```python
from build123d import *

# Parameters (mm, degrees)
EXTRUDE_1_DEPTH     = 0.45
CUT_EXTRUDE_1_DEPTH = 5
SKETCH_4_R          = 0.75
SKETCH_4_R_2        = 0.6
CUT_EXTRUDE_3_DEPTH = 5
EXTRUDE_1_2_DEPTH   = 0.2
EXTRUDE_2_DEPTH     = 0.2


with BuildPart() as part:
    # Эскиз1 → Extrude 1 (new, symmetric)
    with BuildSketch(Plane.XY):
        with BuildLine():
            Line((-11.5, -18.5), (11.5, -18.5))
            Line((11.5, -18.5), (11.5, -6))
            ThreePointArc((11.5, -6), (9.732233047, -5.267766953), (9, -3.5))
            Line((9, -3.5), (5, -3.5))
            Line((5, -3.5), (5, -12))
            Line((5, -12), (-5, -12))
            Line((-5, -12), (-5, -3.5))
            Line((-5, -3.5), (-9, -3.5))
            Line((-9, -3.5), (-11.5, -3.5))
            Line((-11.5, -3.5), (-11.5, -6))
            Line((-11.5, -6), (-11.5, -18.5))
        make_face()
    extrude(amount=EXTRUDE_1_DEPTH, both=True)

    # Эскиз2 → Вырез-Вытянуть1 (cut, symmetric)
    with BuildSketch(Plane.XY):
        Polygon((-0.75, -15.25), (-0.75, -12), (0.75, -12), (0.75, -15.25), (0.75, -15.35), (-0.75, -15.35), align=None)
    extrude(amount=CUT_EXTRUDE_1_DEPTH, both=True, mode=Mode.SUBTRACT)

    # Эскиз4 → Вырез-Вытянуть3 (cut, symmetric)
    with BuildSketch(Plane.XY):
        with Locations((-9.5, -15.5)):
            Circle(SKETCH_4_R)
        with Locations((-2.875, -13.6)):
            Circle(SKETCH_4_R_2)
        with Locations((-7.4, -14.7)):
            Circle(SKETCH_4_R_2)
        with Locations((-7.4, -8.5)):
            Circle(SKETCH_4_R_2)
        with Locations((-7.4, -5)):
            Circle(SKETCH_4_R_2)
        with Locations((7.4, -8.5)):
            Circle(SKETCH_4_R_2)
        with Locations((7.4, -5)):
            Circle(SKETCH_4_R_2)
        with Locations((2.875, -13.6)):
            Circle(SKETCH_4_R_2)
        with Locations((-7.4, -12)):
            Circle(SKETCH_4_R_2)
        with Locations((7.4, -12)):
            Circle(SKETCH_4_R_2)
    extrude(amount=CUT_EXTRUDE_3_DEPTH, both=True, mode=Mode.SUBTRACT)

    # Эскиз5 → Extrude 1 2 (add)
    with BuildSketch(Plane(origin=(0, 0, 0.45), x_dir=(-1, 0, 0), z_dir=(0, 0, -1))):
        Polygon((9.535599533, -15.406551227), (7.435599533, -14.606551227), (7.364400467, -14.793448773), (9.464400467, -15.593448773), align=None)
    extrude(amount=-EXTRUDE_1_2_DEPTH)

    # Эскиз6 → Вытянуть-Тонкостенный2 (add)
    with BuildSketch(Plane(origin=(0, 0, -0.45), x_dir=(-1, 0, 0), z_dir=(0, 0, -1))):
        Polygon((2.847835322, -13.711745605), (7.372835322, -14.811745605), (7.427164678, -14.588254395), (2.902164678, -13.488254395), align=None)
    extrude(amount=EXTRUDE_2_DEPTH)


solid = part.part
```
Source: CAD feature listing. Evaluate the final solid. Frame: model axes, mm. A direction names the side the tool comes from. Coordinates: 2 decimals unless noted, no trailing zeros. Order: outer loops, then holes, each group sorted by start corner. A loop starts at its lowest first (then second) coordinate and runs counter-clockwise, first axis right, second up. Notation, with made-up numbers: (72, 70) - (102, 70) arc R36 cw to (102, 105) - close; hole circle Ø11 at (-8, -17). An arc over 180 degrees is marked (long way). One line per item, written item: value.
1) Cut plane B-B on x = -6.5. Output: boundary loops of the cut face in (y, z), plus the area to 3 significant figures.
Computed values:
outline: (-18.5, -0.45) - (-14.6, -0.45) - (-14.6, -0.65) - (-14.36, -0.65) - (-14.36, -0.45) - (-3.5, -0.45) - (-3.5, 0.45) - (-18.5, 0.45) - close
area: 13.5 mm^2
2) Cut plane C-C on y = -17.25. Output: boundary loops of the cut face in (x, z), plus the area to 3 significant figures.
Computed values:
outline: (-11.5, -0.45) - (11.5, -0.45) - (11.5, 0.45) - (-11.5, 0.45) - close
area: 20.7 mm^2
3) Cut plane A-A on x = 7.4. Output: boundary loops of the cut face in (y, z), plus the area to 3 significant figures.
Computed values:
outline: (-18.5, -0.45) - (-12.6, -0.45) - (-12.6, 0.45) - (-18.5, 0.45) - close; (-11.4, -0.45) - (-9.1, -0.45) - (-9.1, 0.45) - (-11.4, 0.45) - close; (-7.9, -0.45) - (-5.6, -0.45) - (-5.6, 0.45) - (-7.9, 0.45) - close; (-4.4, -0.45) - (-3.5, -0.45) - (-3.5, 0.45) - (-4.4, 0.45) - close
area: 10.3 mm^2
4) Cut plane D-D on x = 4.5. Output: boundary loops of the cut face in (y, z).
Computed values:
outline: (-18.5, -0.45) - (-12, -0.45) - (-12, 0.45) - (-18.5, 0.45) - close
5) Contact query for flat-ended pins moving along their axis: pin 1 (1.4 mm diameter, centred on x = -7.4, y = -12, fed in from -Z); pin 2 (4 mm diameter, centred on x = 4.5, y = -13, fed in from +Z). Output: stop coordinate, or through.
Computed values:
pin 1: stops at z = -0.45
pin 2: stops at z = 0.45
6) Ray query, line 1 (Y direction, x = -7.4, z = -0.2); line 2 (X direction, y = -13.6, z = 0) (3 decimals); line 3 (X direction, y = -9.5, z = 0.25). Return the intervals inside material, ascending. Write a range as [from, to].
Computed values:
line 1: y = [-18.5, -15.3], [-14.1, -12.6], [-11.4, -9.1], [-7.9, -5.6], [-4.4, -3.5]
line 2: x = [-11.5, -3.475], [-2.275, -0.75], [0.75, 2.275], [3.475, 11.5]
line 3: x = [-11.5, -5], [5, 11.5]
7) Reachability of faces 1 (the face through (-3, -12, 0)), 2 (the face through (11.5, -12, 0)) from +Z, -Z, +X, -X, +Y, -Y: full face, straight path, thin tool, end or side. Return the list, or none.
Computed values:
face 1: +Z, -Z, +Y
face 2: +Z, -Z, +X, +Y, -Y
